Read the model definition and answer for the solid it produces. Units are mm, in the model's axes. A direction names the side the tool comes from. Round coordinates to 2 decimals unless told otherwise and drop trailing zeros. Loops run counter-clockwise (first coordinate to the right, second up) from the corner with the lowest first, then second, coordinate; pieces in that order, holes last. Notation, with made-up numbers: M 56.5,38 L 82.5,38 A13 cw 82.5,56 Z; hole C 71.25,52.25 d9. An arc over 180 degrees is marked long. Write each question's results on one line, items separated by ' | '.
from build123d import *

# Parameters (mm, degrees)
PAD_DEPTH = 40
FILLET_R  = 4


with BuildPart() as part:
    # Sketch (on XY_Plane of Origin) → Pad (new body)
    with BuildSketch(Plane.XY):
        Polygon((0, 0), (0, 70), (20, 70), (20, 110), (40, 110), (40, 70), (60, 70), (60, 0), (50, 0), (50, 50), (30, 50), (30, 60), (10, 60), (10, 0), align=None)
    extrude(amount=PAD_DEPTH)

    # Fillet
    fillet_edges = [part.edges().sort_by_distance(p)[0] for p in [
        (0, 0, 20),
        (0, 70, 20),
        (0, 35, 0),
        (0, 35, 40),
        (20, 70, 20),
        (10, 70, 0),
        (10, 70, 40),
        (20, 110, 20),
        (20, 90, 0),
        (20, 90, 40),
        (40, 110, 20),
        (30, 110, 0),
        (30, 110, 40),
        (40, 70, 20),
        (40, 90, 0),
        (40, 90, 40),
        (60, 70, 20),
        (50, 70, 0),
        (50, 70, 40),
        (60, 0, 20),
        (60, 35, 0),
        (60, 35, 40),
        (50, 0, 20),
        (55, 0, 0),
        (55, 0, 40),
        (50, 50, 20),
        (50, 25, 0),
        (50, 25, 40),
        (30, 50, 20),
        (40, 50, 0),
        (40, 50, 40),
        (30, 60, 20),
        (30, 55, 0),
        (30, 55, 40),
        (10, 60, 20),
        (20, 60, 0),
        (20, 60, 40),
        (10, 0, 20),
        (10, 30, 0),
        (10, 30, 40),
        (5, 0, 0),
        (5, 0, 40),
    ]]
    fillet(fillet_edges, radius=FILLET_R)


solid = part.part
Item 1: The part is cut by section B-B (y = 101). Determine the outline of the cut face in (x, z), plus the area to 3 significant figures.
Outcome:
outline: M 20,4 A4 ccw 24,0 L 36,0 A4 ccw 40,4 L 40,36 A4 ccw 36,40 L 24,40 A4 ccw 20,36 Z | area: 786 mm2
Item 2: For faces 4 (the face through (51.141, 25.294, 38.797)), 5 (the face through (21.141, 90.224, 1.203)), 6 (the face through (31.141, 55.014, 1.203)), 7 (the face through (8.859, 1.203, 20.224)), 8 (the face through (50.084, 68.859, 1.203)), determine the directions among +Z, -Z, +X, -X, +Y, -Y from which every point of the face is accessible in a straight line to the end or side of a thin tool.
Outcome:
face 4: +Z, -Y | face 5: -Z, -X, +Y | face 6: -Z, -Y | face 7: +Z, -Z, -Y | face 8: -Z, +X, +Y
Item 3: The part is cut by section A-A (y = 12.5). Determine the outline of the cut face in (x, z).
Outcome:
outline: M 0,4 A4 ccw 4,0 L 6,0 A4 ccw 10,4 L 10,36 A4 ccw 6,40 L 4,40 A4 ccw 0,36 Z; M 50,4 A4 ccw 54,0 L 56,0 A4 ccw 60,4 L 60,36 A4 ccw 56,40 L 54,40 A4 ccw 50,36 Z
Item 4: The part is cut by section C-C (z = 6). Determine the outline of the cut face in (x, y).
Outcome:
outline: M 0,4 A4 ccw 4,0 L 6,0 A4 ccw 10,4 L 10,56 A4 cw 14,60 L 26,60 A4 cw 30,56 L 30,54 A4 ccw 34,50 L 46,50 A4 cw 50,46 L 50,4 A4 ccw 54,0 L 56,0 A4 ccw 60,4 L 60,66 A4 ccw 56,70 L 44,70 A4 cw 40,74 L 40,106 A4 ccw 36,110 L 24,110 A4 ccw 20,106 L 20,74 A4 cw 16,70 L 4,70 A4 ccw 0,66 Z
Item 5: The mould has two halves that part along X. Classify faces 1 (the face through (50, 70, 20)), 2 (the face through (0, 35, 20)), 3 (the face through (31.141, 55.014, 38.797)): pulls with the +X half, pulls with the -X half, needs draft (parallel to the pull), parting line crosses it, or undercut.
Outcome:
face 1: needs draft | face 2: pulls with the -X half | face 3: undercut
Item 6: Flat-ended cylindrical pins translate along their axes: pin 1 (13 mm diameter, centred on x = 23, z = 24.5, fed in from -Y); pin 2 (3.5 mm diameter, centred on x = 50.5, z = 22.5, fed in from +Y); pin 3 (9.5 mm diameter, centred on y = 89, z = 27.5, fed in from +X). Find the tip coordinate at first contact, or state that the pin passes through.
Outcome:
pin 1: stops at y = 57.94 | pin 2: stops at y = 70 | pin 3: stops at x = 40
Item 7: Straight lines are drawn through the part: line 1 (X direction, y = 42.5, z = 24); line 2 (X direction, y = 97, z = 35.5); line 3 (X direction, y = 45.5, z = 3). For each, find the intervals that lie inside material, in ascending order.
Outcome:
line 1: x = 0 to 10, 50 to 60 | line 2: x = 20 to 40 | line 3: x = 0.13 to 9.87, 50.13 to 59.87
